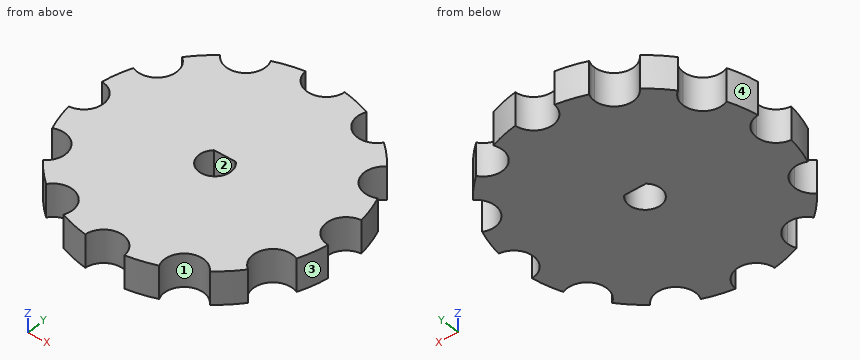
```python
from build123d import *

# Parameters (mm, degrees)
F1_DEPTH = 5
F3_DEPTH = 5.001


with BuildPart() as f1:
    # F0 (on Top) → F1 (new body)
    with BuildSketch(Plane.XY):
        with BuildLine():
            ThreePointArc((19.775, -2.9915506013), (17, 0), (19.775, 2.9915506013))
            ThreePointArc((19.775, 2.9915506013), (19.3185165258, 5.1763809021), (18.6214276605, 7.2967411826))
            ThreePointArc((18.6214276605, 7.2967411826), (14.7224318643, 8.5), (15.6298770592, 12.4782588174))
            ThreePointArc((15.6298770592, 12.4782588174), (14.1421356237, 14.1421356237), (12.4782588174, 15.6298770592))
            ThreePointArc((12.4782588174, 15.6298770592), (8.5, 14.7224318643), (7.2967411826, 18.6214276605))
            ThreePointArc((7.2967411826, 18.6214276605), (5.176380902, 19.3185165258), (2.9915506013, 19.775))
            ThreePointArc((2.9915506013, 19.775), (0, 17), (-2.9915506013, 19.775))
            ThreePointArc((-2.9915506013, 19.775), (-5.176380902, 19.3185165258), (-7.2967411826, 18.6214276605))
            ThreePointArc((-7.2967411826, 18.6214276605), (-7.075125947, 17.9876750517), (-7, 17.3205080757))
            ThreePointArc((-7, 17.3205080757), (-9.1153465233, 14.4539093549), (-12.4782588174, 15.6298770592))
            ThreePointArc((-12.4782588174, 15.6298770592), (-14.1421356237, 14.1421356237), (-15.6298770592, 12.4782588174))
            ThreePointArc((-15.6298770592, 12.4782588174), (-14.6679722089, 11.401446922), (-14.3205080757, 10))
            ThreePointArc((-14.3205080757, 10), (-15.7240680916, 7.4600434301), (-18.6214276605, 7.2967411826))
            ThreePointArc((-18.6214276605, 7.2967411826), (-19.3185165258, 5.1763809021), (-19.775, 2.9915506013))
            ThreePointArc((-19.775, 2.9915506013), (-17.8005682552, 2.0402205763), (-17, 0))
            ThreePointArc((-17, 0), (-17.8005682552, -2.0402205763), (-19.775, -2.9915506013))
            ThreePointArc((-19.775, -2.9915506013), (-19.3185165258, -5.1763809021), (-18.6214276605, -7.2967411826))
            ThreePointArc((-18.6214276605, -7.2967411826), (-15.7240680916, -7.4600434301), (-14.3205080757, -10))
            ThreePointArc((-14.3205080757, -10), (-14.6679722089, -11.401446922), (-15.6298770592, -12.4782588174))
            ThreePointArc((-15.6298770592, -12.4782588174), (-14.1421356237, -14.1421356237), (-12.4782588174, -15.6298770592))
            ThreePointArc((-12.4782588174, -15.6298770592), (-9.1153465233, -14.4539093549), (-7, -17.3205080757))
            ThreePointArc((-7, -17.3205080757), (-7.075125947, -17.9876750517), (-7.2967411826, -18.6214276605))
            ThreePointArc((-7.2967411826, -18.6214276605), (-5.176380902, -19.3185165258), (-2.9915506013, -19.775))
            ThreePointArc((-2.9915506013, -19.775), (0, -17), (2.9915506013, -19.775))
            ThreePointArc((2.9915506013, -19.775), (5.176380902, -19.3185165258), (7.2967411826, -18.6214276605))
            ThreePointArc((7.2967411826, -18.6214276605), (8.5, -14.7224318643), (12.4782588174, -15.6298770592))
            ThreePointArc((12.4782588174, -15.6298770592), (14.1421356237, -14.1421356237), (15.6298770592, -12.4782588174))
            ThreePointArc((15.6298770592, -12.4782588174), (14.7224318643, -8.5), (18.6214276605, -7.2967411826))
            ThreePointArc((18.6214276605, -7.2967411826), (19.3185165258, -5.1763809021), (19.775, -2.9915506013))
        make_face()
    extrude(amount=F1_DEPTH)

    # F2 (on face) → F3 (cut, through all)
    with BuildSketch(Plane.XY.offset(5)):
        with BuildLine():
            Line((1.6522711642, 1.775), (-1.6522711642, 1.775))
            ThreePointArc((-1.6522711642, 1.775), (0, -2.425), (1.6522711642, 1.775))
        make_face()
    extrude(amount=-F3_DEPTH, mode=Mode.SUBTRACT)


solid = f1.part
```
Work out the finished part from the listing and answer in its coordinate system (mm). Face numbers are marked on the shaded views. Round coordinates to 2 decimals unless told otherwise and drop trailing zeros. Write each loop counter-clockwise with the first axis right and the second up, starting at its lowest first coordinate (ties: lowest second). Pieces come first, ordered by that corner, then holes. Notation, with made-up numbers: (45.25, -36.75) - (94.25, -36.75) arc R17 ccw to (94.25, -21.75) - close; hole circle Ø10 at (68.5, -11). An arc over 180 degrees is marked (long way). Return JSON: item names as keys, results as strings. Group by question number.
Q1. The part is cut by section C-C on y = 6. Write down the section's boundary in (x, z).
Q2. The mould has two halves that part along Y. Classify the marked faces 1, 2, 3 and 4: released by +Y, released by -Y, zero draft, split by the parting line, or undercut.
Q3. The part is cut by section B-B on x = 0. Write down the section's boundary in (y, z) (3 decimals), then the cut area to 3 significant figures.
Q4. The part is cut by section D-D on x = 12. Write down the section's boundary in (y, z).
Q5. Each of these flat-tipped pins is pushed along its axis until it touches: pin 1 Ø1.5 at (x, z) = (-1.5, 1.5) entering from +Y; pin 2 Ø2 at (y, z) = (-8.5, 3.5) entering from -X; pin 3 Ø1.5 at (y, z) = (-15, 2) entering from -X. Where does it stop, or does it pass through?
Q6. Find the intervals of material crossed by L1, parallel to X at y = -1.5, z = 1.15; L2, parallel to Y at x = -16, z = 1.6; L3, parallel to Y at x = -2, z = 1.8, in increasing order.
Solved:
{
 "1": {"outline": "(-19.08, 0) - (19.08, 0) - (19.08, 5) - (-19.08, 5) - close"},
 "2": {"face 1": "undercut", "face 2": "undercut", "face 3": "released by -Y", "face 4": "released by +Y"},
 "3": {"outline": "(-17, 0) - (-2.425, 0) - (-2.425, 5) - (-17, 5) - close; (1.775, 0) - (17, 0) - (17, 5) - (1.775, 5) - close", "area": "149 mm²"},
 "4": {"outline": "(-15.08, 0) - (15.08, 0) - (15.08, 5) - (-15.08, 5) - close"},
 "5": {"pin 1": "y = 18.02", "pin 2": "x = -15.66", "pin 3": "x = -14.03"},
 "6": {"L1": "-17.4 to -1.91, 1.91 to 17.4", "L2": "-7.31 to 7.31", "L3": "-17.76 to -1.37, 1.37 to 17.76"}
}
